Autodesk Inventor part; units mm, degrees
ref_plane "Work Plane1" through (40, 0, 0) normal (-1, 0, 0) x (0, 0, 1)
ref_plane "YZ Plane" through (0, 0, 0) normal (1, 0, 0) x (0, 1, 0)
ref_plane "XZ Plane" through (0, 0, 0) normal (0, 1, 0) x (-1, 0, 0)
sketch "Sketch2" plane through (0, 0, 0) normal (1, 0, 0) x (0, 1, 0)
  line L0 (0, 0) -> (50, 0)
  line L1 (50, 0) -> (50, -50)
  line L2 (50, -50) -> (0, -50)
  line L3 (0, -50) -> (0, 0)
  line L4 (0, 0) -> (40, 0)
  line L5 (40, 0) -> (40, -40)
  line L6 (40, -40) -> (0, -40)
  line L7 (0, -40) -> (0, 0)
  dimension "d5" = 50
  dimension "d6" = 50
  dimension "d7" = 10
  dimension "d8" = 10
extrude "Extrusion1" add sketch "Sketch2" along normal blind 80 contours L0 L1 L2 L3 L6 L5
fillet "Fillet1" radius 2 2 edges at (40, 40, -40) (40, 50, -50)
sketch "Sketch6" plane through (0, 0, 0) normal (-1, 0, 0) x (0, 0, 1)
  line L0 (-40, 0) -> (-50, 0)
  line L1 (-45, 0) -> (-45, 50)
  line L2 (-48, 50) -> (0, 50)
  line L3 (0, 50) -> (0, 40)
  line L4 (0, 45) -> (-50, 45)
  point P0 (0, 0)
  point P1 (-50, 50)
  point P2 (-5, 45)
  point P3 (-20, 45)
  point P4 (-35, 45)
  point P5 (-45, 35)
  point P6 (-45, 5)
  point P7 (-45, 20)
  dimension "d23" = 5
  dimension "d25" = 20
  dimension "d26" = 35
  dimension "d27" = 5
  dimension "d28" = 20
  dimension "d29" = 35
hole "Hole1" at (0, 45, -5) at (0, 45, -20) at (0, 45, -35) at (0, 35, -45) at (0, 5, -45) at (0, 20, -45) direction (1, 0, 0) diameter 4.917 depth 17.1 tip angle 118
ref_plane "Work Plane1" through (40, 0, 0) normal (-1, 0, 0) x (0, 0, 1)
mirror "Mirror1" about plane through (40, 0, 0) normal (-1, 0, 0) of "Hole1"
ref_plane "Work Plane2" through (40, 0, 0) normal (-1, 0, 0) x (0, 0, 1)
properties part number "Profile_Middle_02"
Read the model definition and answer for the solid it produces. Units are mm, in the model's axes. A direction names the side the tool comes from. Give positions to 0.01 mm unless a question says otherwise; leave off trailing zeros. Write each loop counter-clockwise with the first axis right and the second up, starting at its lowest first coordinate (ties: lowest second). Pieces come first, ordered by that corner, then holes. Notation, with made-up numbers: (38.25, 69) - (87.25, 69) arc R26 ccw to (87.25, 93) - close; hole circle Ø4 at (-14.5, 3). An arc over 180 degrees is marked (long way). Write item = value, one per line. Start each with the question number.
Item 1: Find the intervals of material crossed by probe 1 along Y at (x, z) = (13, -45); probe 2 along Z at (x, y) = (8, 5); probe 3 along Y at (x, z) = (6.5, -5), in increasing order. Write a range as [from, to].
Item 2: Each of these flat-tipped pins is pushed along its axis until it touches: P1, Ø4.5, axis at y = 45, z = -20, coming from the +X side; P2, Ø2, axis at x = 13.5, y = 17.5, coming from the +Z side; P3, Ø3, axis at y = 38, z = -15.5, coming from the -X side; P4, Ø4, axis at y = 20, z = -45, coming from the -X side. Where does it stop, or does it pass through?
Item 3: Find section C-C (z = -31). Give the vertices of the cut face in (x, y), then the cut area to 3 significant figures.
Item 4: The mould has two halves that part along Y. Classify faces 5 (the conical face through (18.32, 5.29, -45.31)), 6 (the flat face through (39, 50, -24)), 7 (the flat face through (39, 0, -45)): +Y half, -Y half, draft (parallel to the pull), parting line (faces both ways), or undercut.
Item 5: A tool of negligible diameter and unlimited length cuts with its end or side. For faces 1 (the flat face through (39, 40, -19)), 2 (the flat face through (0, 34, -42)), 3 (the cylindrical face through (71.33, 34.06, -42.73)), 4 (the cylindrical face through (8.67, 45.94, -32.73)), from which of +Z, -Z, +X, -X, +Y, -Y can it reach the whole face along a straight path? Write none if from no direction.
Item 6: Find section A-A (x = 73). Give the vertices of the cut face in (y, z), then the cut area to 3 significant figures.
Item 7: Find section B-B (x = 21.5). Give the vertices of the cut face in (y, z), then the cut area to 3 significant figures.
Response:
q1.probe_1 = [0, 2.54], [7.46, 17.54], [22.46, 32.54], [37.46, 50]
q1.probe_2 = [-50, -47.46], [-42.54, -40]
q1.probe_3 = [40, 42.54], [47.46, 50]
q2.P1 = 62.77
q2.P2 = -40
q2.P3 = through
q2.P4 = 17.38
q3.outline = (0, 40) - (80, 40) - (80, 50) - (0, 50) - close
q3.area = 800 mm²
q4.face_5 = undercut
q4.face_6 = +Y half
q4.face_7 = -Y half
q5.face_1 = +Z, +X, -X, -Y
q5.face_2 = +Z, -Z, -X, +Y, -Y
q5.face_3 = +X
q5.face_4 = -X
q6.outline = (0, -50) - (48, -50) arc R2 ccw to (50, -48) - (50, 0) - (40, 0) - (40, -38) arc R2 cw to (38, -40) - (0, -40) - close; hole circle Ø4.92 at (5, -45); hole circle Ø4.92 at (20, -45); hole circle Ø4.92 at (35, -45); hole circle Ø4.92 at (45, -35); hole circle Ø4.92 at (45, -20); hole circle Ø4.92 at (45, -5)
q6.area = 786 mm²
q7.outline = (0, -50) - (48, -50) arc R2 ccw to (50, -48) - (50, 0) - (40, 0) - (40, -38) arc R2 cw to (38, -40) - (0, -40) - close
q7.area = 900 mm²
